CAD build for the part. Positions are in the model's coordinates, mm. A direction names the side the tool comes from. Round coordinates to 2 decimals unless told otherwise and drop trailing zeros. Order: outer loops, then holes, each group sorted by start corner. A loop starts at its lowest first (then second) coordinate and runs counter-clockwise, first axis right, second up. Notation, with made-up numbers: M -9,74 L 13,74 A30 cw 13,105 Z; hole C 37.25,60.5 d5. An arc over 180 degrees is marked long. Put each result on its own line as item: value.
```python
from build123d import *

# Parameters (mm, degrees)
SKETCH1_R           = 17.653
BOSS_EXTRUDE1_DEPTH = 7.62
SKETCH2_R           = 5.969
BOSS_EXTRUDE2_DEPTH = 6.35
CHAMFER1_SIZE       = 10
CHAMFER1_SIZE2      = 3.639702343
FILLET1_R           = 1.524
FILLET2_R           = 0.508


with BuildPart() as part:
    # Sketch1 → Boss-Extrude1 (new body)
    with BuildSketch(Plane(origin=(0, 0, 0), x_dir=(1, 0, 0), z_dir=(0, 1, 0))):
        with Locations(Location((0, 0, 0), (0, 0, 90))):
            Circle(SKETCH1_R)
    extrude(amount=BOSS_EXTRUDE1_DEPTH)

    # Sketch2 → Boss-Extrude2 (add)
    with BuildSketch(Plane(origin=(0, 7.62, 0), x_dir=(1, 0, 0), z_dir=(0, 1, 0))):
        with Locations(Location((0, 0, 0), (0, 0, 270))):
            Circle(SKETCH2_R)
    extrude(amount=BOSS_EXTRUDE2_DEPTH)

    # Chamfer1
    chamfer1_edges = [part.edges().sort_by_distance(p)[0] for p in [
        (0, 0, 17.653),
    ]]
    chamfer1_side = [part.faces().sort_by_distance(p)[0] for p in [
        (0, 0, 0),
    ]]
    chamfer(chamfer1_edges, length=CHAMFER1_SIZE, length2=CHAMFER1_SIZE2, reference=chamfer1_side[0])

    # Fillet1
    fillet1_edges = [part.edges().sort_by_distance(p)[0] for p in [
        (0, 0, 7.653),
        (0, 3.639702343, 17.653),
    ]]
    fillet(fillet1_edges, radius=FILLET1_R)

    # Fillet2
    fillet2_edges = [part.edges().sort_by_distance(p)[0] for p in [
        (0, 13.97, -5.969),
    ]]
    fillet(fillet2_edges, radius=FILLET2_R)


solid = part.part
```
Item 1: Band-saw the part on A-A on y = 10. Give the cut face in (x, z), and give its area (3 significant figures).
Answers below:
outline: C 0,0 d11.94
area: 112 mm²
Item 2: Pin check, flat tips, straight feed: P1, Ø3, axis at x = -2, z = 8.5, coming from the +Y side; P2, Ø3, axis at x = -8.5, y = 11, coming from the +Z side; P3, Ø1, axis at y = 9, z = -3, coming from the +X side. Stop position of each tip, or through.
Answers below:
P1: y = 7.62
P2: through
P3: x = 5.42
Item 3: Probe line 1 along Z through (x, y) = (-15, 5); line 2 along Y through (x, z) = (12, 12); line 3 along X through (y, z) = (11.5, -4). List the from-to ranges inside material, lowest first. Write a range as [from, to].
Answers below:
line 1: [-9.31, 9.31]
line 2: [3.44, 7.62]
line 3: [-4.43, 4.43]
Item 4: Tool access for faces 1 (the cylindrical face through (1.793, 10.5, 5.693)), 2 (the flat face through (0, 0, 0)): list every direction of +Z, -Z, +X, -X, +Y, -Y with a clear straight run to the whole face (end or side of a thin tool).
Answers below:
face 1: +Y
face 2: +Z, -Z, +X, -X, -Y
